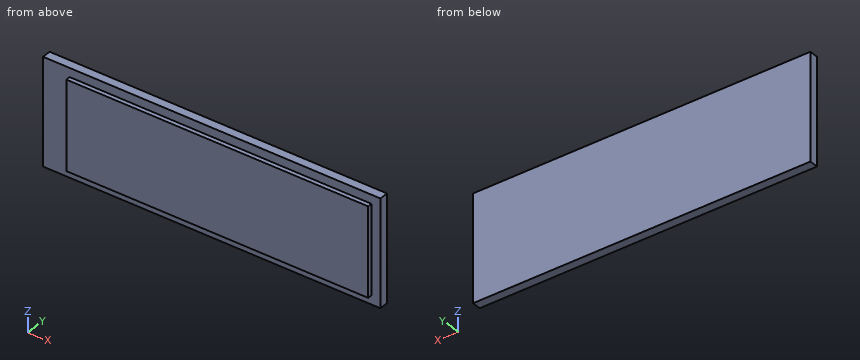
from build123d import *

# Parameters (mm, degrees)
BOX_W        = 38
BOX_H        = 1
BOX_DEPTH    = 12
BOX001_W     = 34
BOX001_H     = 1
BOX001_DEPTH = 10


with BuildPart() as cubo:
    # Box → Box (new body)
    with BuildSketch(Plane.XY):
        with Locations((19, 0.5)):
            Rectangle(BOX_W, BOX_H)
    extrude(amount=BOX_DEPTH)


with BuildPart() as display:
    # Box001 → Box001 (new body)
    with BuildSketch(Plane(origin=(3, -0.5, 1), x_dir=(1, 0, 0), z_dir=(0, 0, 1))):
        with Locations((17, 0.5)):
            Rectangle(BOX001_W, BOX001_H)
    extrude(amount=BOX001_DEPTH)

    # Fusion: union Cubo
    add(cubo.part)


solid = display.part
Source: CAD feature listing. Evaluate the final solid. Frame: model axes, mm. Give positions to 0.01 mm unless a question says otherwise; leave off trailing zeros. Write each loop counter-clockwise with the first axis right and the second up, starting at its lowest first coordinate (ties: lowest second). Pieces come first, ordered by that corner, then holes. Notation, with made-up numbers: M 44,6.25 L 85,6.25 A20 cw 85,23.25 Z; hole C -36.75,33 d10. An arc over 180 degrees is marked long. Return JSON: item names as keys, results as strings. Group by question number.
1) Cut plane C-C, the plane y = -0.25. Output: boundary loops of the cut face in (x, z), plus the area to 3 significant figures.
2) Cut plane B-B, the plane x = 5. Output: boundary loops of the cut face in (y, z).
3) Material intervals for line 1 along Z through (x, y) = (33, -0.1); line 2 along X through (y, z) = (-0.2, 8.25); line 3 along Y through (x, z) = (17, 11.5), sorted ascending. Write a range as [from, to].
4) Cut plane A-A, the plane z = 5.75. Output: boundary loops of the cut face in (x, y).
Recorded:
{
 "1": {"outline": "M 3,1 L 37,1 L 37,11 L 3,11 Z", "area": "340 mm²"},
 "2": {"outline": "M -0.5,1 L 0,1 L 0,0 L 1,0 L 1,12 L 0,12 L 0,11 L -0.5,11 Z"},
 "3": {"line 1": "z = [1, 11]", "line 2": "x = [3, 37]", "line 3": "y = [0, 1]"},
 "4": {"outline": "M 0,0 L 3,0 L 3,-0.5 L 37,-0.5 L 37,0 L 38,0 L 38,1 L 0,1 Z"}
}
